Check sheet for the drawn part. Datum: minimum x, y, z corner. Units: mm. A direction names the side the tool comes from. Coordinates: 2 decimals unless noted, no trailing zeros. Order: outer loops, then holes, each group sorted by start corner. A loop starts at its lowest first (then second) coordinate and runs counter-clockwise, first axis right, second up.
1. Thickness scan on line 1 (Z direction, x = 25.4, y = 3.55); line 2 (X direction, y = 2.4, z = 26); line 3 (Z direction, x = 3.5, y = 0.5). Record the ranges inside material, lowest first.
2. Set-up check for the marked faces 4 and 5: record each of +Z, -Z, +X, -X, +Y, -Y from which the full face is reachable in a straight line by a thin tool's end or side.
3. Draft check along X on the marked faces 1, 2 and 3. Enter one of: released by +X, released by -X, zero draft, split by the parting line, or undercut.
4. Cross-section at D-D (z = 7). Enter the section's corners in (x, y), then the cut area to 3 significant figures.
5. Gauge pin test, flat ends, axial feed: pin 1 Ø2 at (x, y) = (36, 2.5) entering from -Z; pin 2 Ø2 at (y, z) = (2, 42.5) entering from +X; pin 3 Ø2 at (y, z) = (1.5, 7.5) entering from -X. Record the tip position at first contact, or that the pin passes through.
6. Cross-section at C-C (z = 20.5). Enter the section's corners in (x, y).
7. Cross-section at B-B (y = 0.85). Enter the section's corners in (x, z) (3 decimals).
8. Cross-section at A-A (x = 25.4). Enter the section's corners in (y, z).
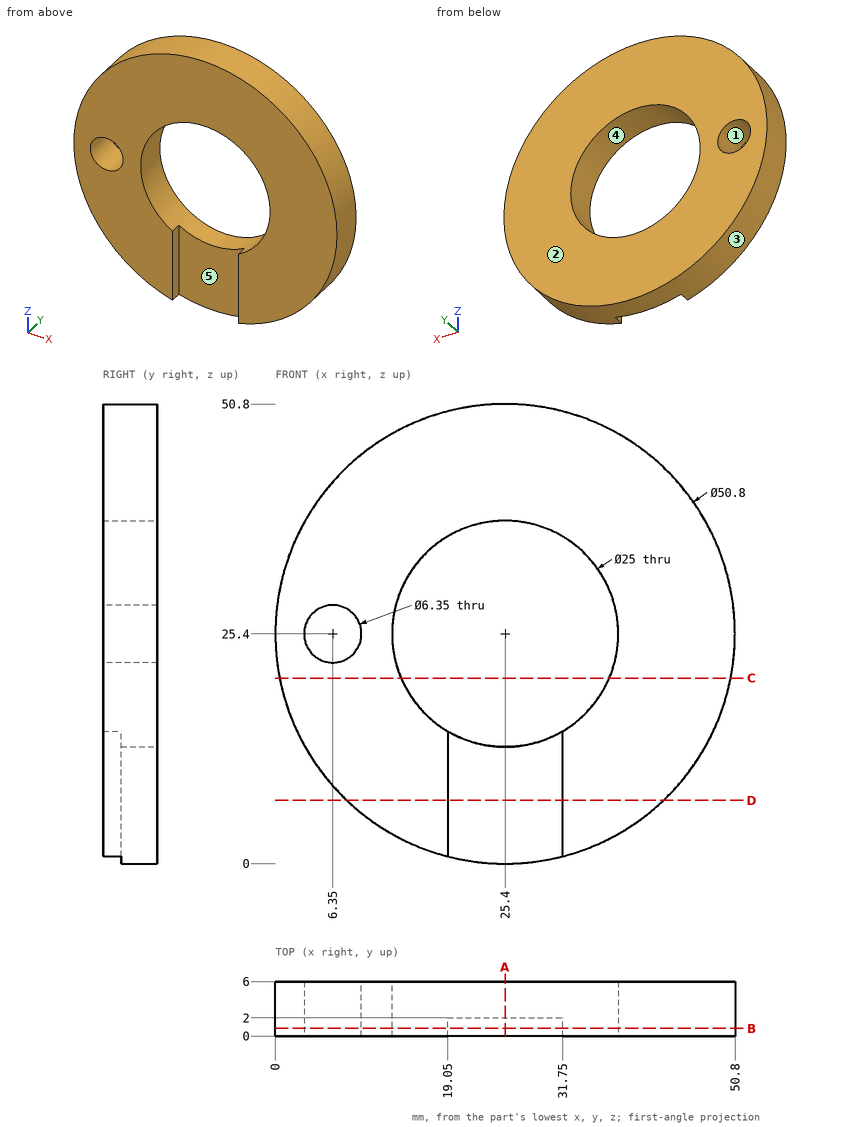
Data:
1. line 1: z = 0 to 12.9, 37.9 to 50.8
1. line 2: x = 0.01 to 3.23, 9.47 to 12.91, 37.89 to 50.79
1. line 3: z = 12.53 to 24, 26.8 to 38.27
2. face 4: +Y, -Y
2. face 5: -Z, -Y
3. face 1: undercut
3. face 2: zero draft
3. face 3: split by the parting line
4. outline: (7.89, 0) - (19.05, 0) - (19.05, 2) - (31.75, 2) - (31.75, 0) - (42.91, 0) - (42.91, 6) - (7.89, 6) - close
4. area: 185 mm2
5. pin 1: stops at z = 1.88
5. pin 2: stops at x = 45.05
5. pin 3: stops at x = 6.44
6. outline: (0.48, 0) - (13.9, 0) - (13.9, 6) - (0.48, 6) - close; (36.9, 0) - (50.32, 0) - (50.32, 6) - (36.9, 6) - close
7. outline: (19.05, 0.807) - (19.05, 14.633) arc R12.5 cw (long way) to (31.75, 14.633) - (31.75, 0.807) arc R25.4 ccw (long way) to start; hole circle Ø6.35 at (6.35, 25.4)
8. outline: (0, 37.9) - (6, 37.9) - (6, 50.8) - (0, 50.8) - close; (2, 0) - (6, 0) - (6, 12.9) - (2, 12.9) - close
